Job drawing, mm, ordinate dimensions from the low corner. One solid piece. Round coordinates to 2 decimals unless told otherwise and drop trailing zeros. Loops run counter-clockwise (first coordinate to the right, second up) from the corner with the lowest first, then second, coordinate; pieces in that order, holes last. Notation, with made-up numbers: M -10,-33 L 10,-33 A12 ccw 10,-27 Z; hole C 65.25,-24 d5. An arc over 180 degrees is marked long. Use a Markdown table: item, result. Add a question column.
(1) Band-saw the part on A-A, the plane x = 0.5. Write the cut outline in (y, z) (1 decimal).
(2) Flat gauge pins, fed straight in: P1, Ø0.6, axis at x = 3, y = 0.5, coming from the +Z side; P2, Ø0.6, axis at x = 0.5, z = 5, coming from the -Y side; P3, Ø0.6, axis at x = 0.5, y = 0.5, coming from the -Z side (1 decimal). Where does each tip first touch, or does it go through?
(3) Band-saw the part on B-B, the plane z = 3.25. Write the cut outline in (x, y) (1 decimal).
(4) Wall check: L1, parallel to Z at x = 3, y = 0.9 (1 decimal); L2, parallel to X at y = 0.05, z = 1.5 (1 decimal). Give the ranges that are in metal, low to high.
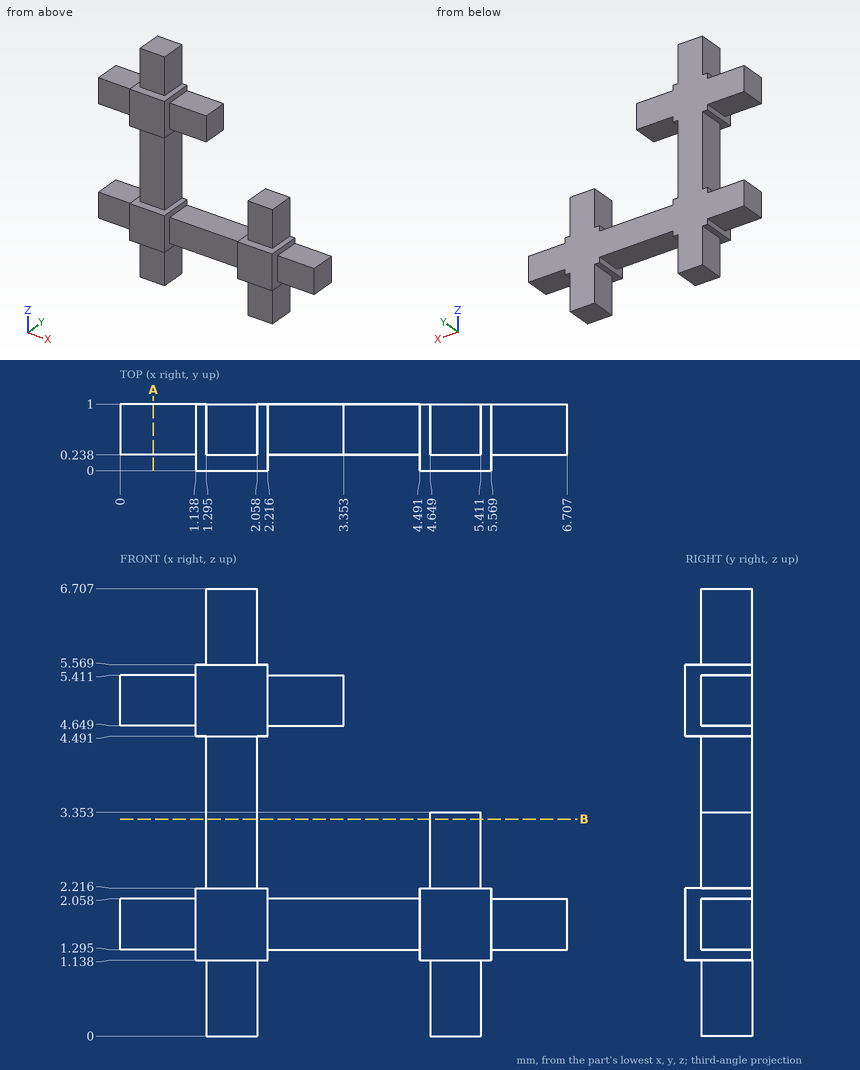
Return value:
| question | item | result |
|---|---|---|
| 1 | outline | M 0.2,1.3 L 1,1.3 L 1,2.1 L 0.2,2.1 Z; M 0.2,4.6 L 1,4.6 L 1,5.4 L 0.2,5.4 Z |
| 2 | P1 | z = 5.41 |
| 2 | P2 | y = 0.24 |
| 2 | P3 | z = 1.3 |
| 3 | outline | M 1.3,0.2 L 2.1,0.2 L 2.1,1 L 1.3,1 Z; M 4.6,0.2 L 5.4,0.2 L 5.4,1 L 4.6,1 Z |
| 4 | L1 | 1.3 to 2.1, 4.6 to 5.4 |
| 4 | L2 | 1.1 to 2.2, 4.5 to 5.6 |
